Source: CAD feature listing. Evaluate the final solid. Frame: model axes, mm. A direction names the side the tool comes from. Give positions to 0.01 mm unless a question says otherwise; leave off trailing zeros. Order: outer loops, then holes, each group sorted by start corner. A loop starts at its lowest first (then second) coordinate and runs counter-clockwise, first axis right, second up.
from build123d import *

# Parameters (mm, degrees)
F0_R     = 33.455584
F1_DEPTH = 25.4
F2_R     = 5.08
F3_R     = 5.08
F4_W     = 27.818047
F4_H     = 23.049239
F5_DEPTH = 25.401
F7_DEPTH = 25.401


with BuildPart() as f1:
    # F0 (on Front) → F1 (new body)
    with BuildSketch(Plane.XZ):
        Circle(F0_R)
    extrude(amount=F1_DEPTH)

    # F2
    f2_edges = [f1.edges().sort_by_distance(p)[0] for p in [
        (-33.455584, -25.4, 0),
    ]]
    fillet(f2_edges, radius=F2_R)

    # F3
    f3_edges = [f1.edges().sort_by_distance(p)[0] for p in [
        (-33.455584, 0, 0),
    ]]
    fillet(f3_edges, radius=F3_R)

    # F4 (on face) → F5 (cut, through all)
    with BuildSketch(Plane.XZ.offset(25.4)):
        with Locations((0.132467, 3.83878)):
            Rectangle(F4_W, F4_H)
    extrude(amount=-F5_DEPTH, mode=Mode.SUBTRACT)

    # F6 (on face) → F7 (cut, through all)
    with BuildSketch(Plane.XZ.offset(25.4)):
        Polygon((-13.776556, -7.685839), (-21.724571, -10.60011), (20.3999, -12.454647), (14.041491, -7.685839), align=None)
    extrude(amount=-F7_DEPTH, mode=Mode.SUBTRACT)


solid = f1.part
1) Reachability of faces 1 (the face through (0, 0, -12)), 2 (the face through (-0.957, -12.878, -11.514)) from +Z, -Z, +X, -X, +Y, -Y: full face, straight path, thin tool, end or side. Return the list, or none.
Checks:
face 1: +Z, -Z, +X, -X, +Y
face 2: +Y, -Y
2) Section query C-C on y = -7. Output: boundary loops of the cut face in (x, z), and give its area (3 significant figures).
Checks:
outline: circle Ø66.91 at (0, 0); hole (-21.72, -10.6) - (20.4, -12.45) - (14.04, -7.69) - (14.04, 15.36) - (-13.78, 15.36) - (-13.78, -7.69) - close
area: 2,740 mm2
3) Section query B-B on x = 0. Output: boundary loops of the cut face in (y, z).
Checks:
outline: (-25.4, -28.38) arc R5.08 ccw to (-20.32, -33.46) - (-5.08, -33.46) arc R5.08 ccw to (0, -28.38) - (0, -11.56) - (-25.4, -11.56) - close; (-25.4, 15.36) - (0, 15.36) - (0, 28.38) arc R5.08 ccw to (-5.08, 33.46) - (-20.32, 33.46) arc R5.08 ccw to (-25.4, 28.38) - close
4) Section query A-A on z = 0. Output: boundary loops of the cut face in (x, y), and give its area (3 significant figures).
Checks:
outline: (-33.46, -20.32) arc R5.08 ccw to (-28.38, -25.4) - (-13.78, -25.4) - (-13.78, 0) - (-28.38, 0) arc R5.08 ccw to (-33.46, -5.08) - close; (14.04, -25.4) - (28.38, -25.4) arc R5.08 ccw to (33.46, -20.32) - (33.46, -5.08) arc R5.08 ccw to (28.38, 0) - (14.04, 0) - close
area: 971 mm2
5) First-contact query: pin 1 Ø10 at (y, z) = (-16.5, 15.5) entering from +X; pin 2 Ø2 at (x, y) = (-5.5, -21) entering from +Z; pin 3 Ø3 at (y, z) = (-14.5, -9.5) entering from -X (3 decimals). Flat tips, straight axial feed; report the tip coordinate or a pass-through.
Checks:
pin 1: stops at x = 31.77
pin 2: stops at z = 33.13
pin 3: stops at x = -32.485
6) Pull-direction query (X, two-part tool) for faces 3 (the face through (-13.777, -13, 4)), 4 (the face through (0, -25.4, -12)), 5 (the face through (17.265, -12.878, -10.104)), 6 (the face through (-26.549, -12.593, -20.357)); classes: +X half, -X half, draft (parallel to the pull), parting line (faces both ways), or undercut.
Checks:
face 3: undercut
face 4: draft
face 5: undercut
face 6: parting line
7) Ray query, L1, parallel to Z at x = -11.5, y = -9; L2, parallel to Z at x = 11.5, y = -5; L3, parallel to X at y = -15.5, z = 5. Return the intervals inside material, ascending.
Checks:
L1: z = -31.42 to -11.05, 15.36 to 31.42
L2: z = -31.42 to -12.06, 15.36 to 31.42
L3: x = -33.08 to -13.78, 14.04 to 33.08
